```python
from build123d import *

# Parameters (mm, degrees)
F1_DEPTH = 12.7
F2_R     = 1.651
F3_DEPTH = 3.175
F4_R     = 6.34999


# Not quite as in the source:
# - a fillet or chamfer is up to 0.001 mm smaller than in the source, because OpenCascade refuses the exact size


with BuildPart() as f1:
    # F0 (on Top) → F1 (new body)
    with BuildSketch(Plane.XY):
        Polygon((0, -12.5), (3, -12.5), (3, -2.5), (26, -2.5), (26, 0), (0, 0), align=None)
    extrude(amount=F1_DEPTH)

    # F2 (on face) → F3 (cut)
    with BuildSketch(Plane.XZ.offset(2.5)):
        with Locations((20, 6.35)):
            Circle(F2_R)
    extrude(amount=-F3_DEPTH, mode=Mode.SUBTRACT)

    # F4 (radius 6.35 in the source; OpenCascade refuses exactly that, so slightly less here)
    f4_edges = [f1.edges().sort_by_distance(p)[0] for p in [
        (26, -1.25, 12.7),
        (26, -1.25, 0),
    ]]
    fillet(f4_edges, radius=F4_R)


solid = f1.part
```
The listing builds one solid part. Answer for the finished solid, in the listing's coordinates (mm). A direction names the side the tool comes from. Give positions to 0.01 mm unless a question says otherwise; leave off trailing zeros. Loops run counter-clockwise (first coordinate to the right, second up) from the corner with the lowest first, then second, coordinate; pieces in that order, holes last. Notation, with made-up numbers: M 0.25,42.25 L 17.25,42.25 A31 cw 17.25,77.25 Z; hole C 82.25,-6.75 d2. An arc over 180 degrees is marked long. One line per item, written item: value.
Q1. Find the intervals of material crossed by line 1 (Y direction, x = 19.75, z = 2); line 2 (X direction, y = -4, z = 7); line 3 (Z direction, x = 20, y = -1.75), in increasing order. Write a range as from..to.
Working result:
line 1: y = -2.5..0
line 2: x = 0..3
line 3: z = 0.01..4.7, 8..12.69
Q2. Determine the mould class of faces 3 (the face through (6, -2, 12.7)), 4 (the face through (20, -1, 8)), 5 (the face through (6, -2, 0)), 6 (the face through (14, -2.5, 6)) for opening direction Z: +Z half, -Z half, draft (parallel to the pull), parting line (faces both ways), or undercut.
Working result:
face 3: +Z half
face 4: undercut
face 5: -Z half
face 6: draft
Q3. A cutting plane is placed at C-C on z = 2.75. Determine the outline of the cut face in (x, y), then the cut area to 3 significant figures.
Working result:
outline: M 0,-12.5 L 3,-12.5 L 3,-2.5 L 24.88,-2.5 L 24.88,0 L 0,0 Z
area: 92.2 mm^2
Q4. A cutting plane is placed at D-D on y = -11.5. Determine the outline of the cut face in (x, z).
Working result:
outline: M 0,0 L 3,0 L 3,12.7 L 0,12.7 Z
Q5. Flat-ended cylindrical pins translate along their axes: P1, Ø1.5, axis at x = 13, z = 2.5, coming from the -Y side; P2, Ø3, axis at x = 20, z = 6.35, coming from the -Y side; P3, Ø5, axis at y = -8, z = 3.5, coming from the +X side. Find the tip coordinate at first contact, or state that the pin passes through.
Working result:
P1: stops at y = -2.5
P2: passes through
P3: stops at x = 3
Q6. A cutting plane is placed at B-B on x = 20. Determine the outline of the cut face in (y, z), then the cut area to 3 significant figures.
Working result:
outline: M -2.5,0.01 L 0,0.01 L 0,4.7 L -2.5,4.7 Z; M -2.5,8 L 0,8 L 0,12.69 L -2.5,12.69 Z
area: 23.4 mm^2
Q7. For faces 1 (the face through (3, -8, 6)), 2 (the face through (13, 0, 6)), determine the directions among +Z, -Z, +X, -X, +Y, -Y from which every point of the face is accessible in a straight line to the end or side of a thin tool.
Working result:
face 1: +Z, -Z, +X, -Y
face 2: +Z, -Z, +X, -X, +Y
